Source: CAD feature listing. Evaluate the final solid. Frame: model axes, mm. Round coordinates to 2 decimals unless told otherwise and drop trailing zeros. Loops run counter-clockwise (first coordinate to the right, second up) from the corner with the lowest first, then second, coordinate; pieces in that order, holes last. Notation, with made-up numbers: M -15,83.25 L 38,83.25 A23 cw 38,122.25 Z; hole C 50.5,-35.5 d10. An arc over 180 degrees is marked long. Write each question's results on one line, items separated by ' | '. Start each with the question number.
1. Section B-B on y = 116. Output: boundary loops of the cut face in (x, z), and give its area (3 significant figures).
2. Ray query, line 1 (Z direction, x = 1.3, y = 138); line 2 (Y direction, x = 3.1, z = 18.5); line 3 (Z direction, x = 3.65, y = 124). Return the intervals inside material, ascending.
3. Section D-D on z = -47.5. Output: boundary loops of the cut face in (x, y).
4. Section C-C on y = 65.5. Output: boundary loops of the cut face in (x, z).
5. Contact query for flat-ended pins moving along their axis: pin 1 Ø2 at (x, z) = (3, -0.5) entering from -Y; pin 2 Ø1.5 at (x, y) = (2.5, 65.5) entering from -Z; pin 3 Ø1.5 at (x, z) = (1.5, 86) entering from -Y. Output: stop coordinate, or through.
6. Section A-A on x = 2.5. Output: boundary loops of the cut face in (y, z).
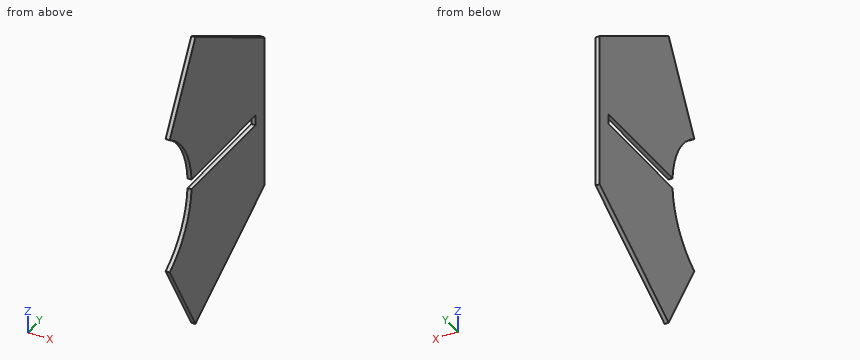
from build123d import *

# Parameters (mm, degrees)
BOSS_EXTRU_1_DEPTH = 4


with BuildPart() as part:
    # Esquisse1 → Boss.-Extru.1 (new body)
    with BuildSketch(Plane(origin=(0, 0, 0), x_dir=(0, 0, -1), z_dir=(1, 0, 0))):
        with BuildLine():
            Line((-68.416006899, 39.5), (-148.5, 85.736514975))
            Line((-148.5, 85.736514975), (-76.75644347, 210))
            Line((-76.75644347, 210), (76.75644347, 210))
            Line((76.75644347, 210), (148.5, 85.736514975))
            Line((148.5, 85.736514975), (68.416006899, 39.5))
            ThreePointArc((68.416006899, 39.5), (41.646346215, 67.13107959), (5, 78.841613378))
            Line((5, 78.841613378), (5, 193.841613378))
            Line((5, 193.841613378), (-5, 193.841613378))
            Line((-5, 193.841613378), (-5, 78.841613378))
            ThreePointArc((-5, 78.841613378), (-41.646346215, 67.13107959), (-68.416006899, 39.5))
        make_face()
    extrude(amount=BOSS_EXTRU_1_DEPTH)


solid = part.part
Taken from the geometry:
1) outline: M 0,-131.03 L 4,-131.03 L 4,-5 L 0,-5 Z; M 0,5 L 4,5 L 4,131.03 L 0,131.03 Z | area: 1,010 mm^2
2) line 1: -118.33 to -5, 5 to 118.33 | line 2: 76.8 to 210 | line 3: -126.41 to -5, 5 to 126.41
3) outline: M 0,63.12 L 4,63.12 L 4,210 L 0,210 Z
4) outline: M 0,-113.45 L 4,-113.45 L 4,-44.17 L 0,-44.17 Z; M 0,44.17 L 4,44.17 L 4,113.45 L 0,113.45 Z
5) pin 1: y = 193.84 | pin 2: z = -114.75 | pin 3: y = 49.22
6) outline: M 39.5,-68.42 L 85.74,-148.5 L 210,-76.76 L 210,76.76 L 85.74,148.5 L 39.5,68.42 A79 cw 78.84,5 L 193.84,5 L 193.84,-5 L 78.84,-5 A79 cw Z
